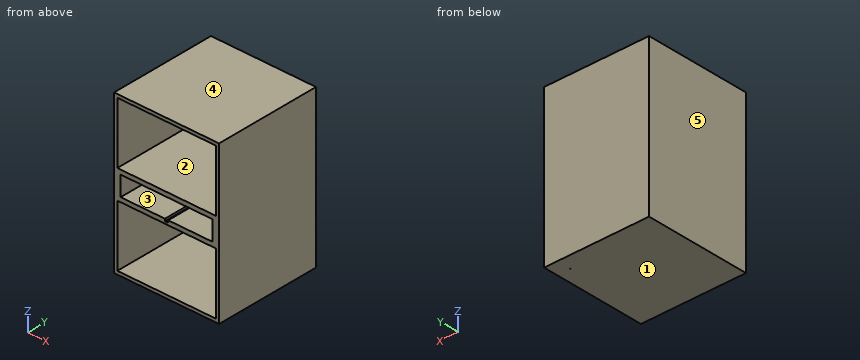
from build123d import *

# Parameters (mm, degrees)
F0_W     = 1219.2
F0_H     = 1828.8
F0_W_2   = 1143
F0_H_2   = 711.2
F0_W_3   = 1066.8
F0_H_3   = 228.6
F1_DEPTH = 609.6
F2_W     = 1219.2
F2_H     = 1828.8
F3_DEPTH = 12.7
F5_D     = 2.54
F7_D     = 2.54
F7_DEPTH = 12.7
F7_TIP   = 0.7630929862
F8_W     = 38.1
F8_H     = 1219.2
F9_DEPTH = 25.4


# Not quite as in the source:
# - a feature names something its author has since deleted; it is built from what else it names


with BuildPart() as f1:
    # F0 (on Front) → F1 (new body, symmetric)
    with BuildSketch(Plane.XZ):
        Rectangle(F0_W, F0_H)
        with Locations((0, -520.7)):
            Rectangle(F0_W_2, F0_H_2, mode=Mode.SUBTRACT)
        Rectangle(F0_W_3, F0_H_3, mode=Mode.SUBTRACT)
        with Locations((0, 520.7)):
            Rectangle(F0_W_2, F0_H_2, mode=Mode.SUBTRACT)
    extrude(amount=F1_DEPTH, both=True)

    # F2 (on face) → F3 (join)
    with BuildSketch(Plane(origin=(0, 609.6, 0), x_dir=(-1, 0, 0), z_dir=(0, 1, 0))):
        Rectangle(F2_W, F2_H)
    extrude(amount=F3_DEPTH)

    # F5 (through all)
    with Locations(Plane(origin=(-609.6, 0, 0), x_dir=(0, -1, 0), z_dir=(-1, 0, 0))):
        with Locations((-400.05, 685.8), (-311.15, 685.8), (311.15, 685.8), (400.05, 685.8)):
            Hole(F5_D / 2)

    # F7
    with Locations(Plane(origin=(0, 0, -914.4), x_dir=(1, 0, 0), z_dir=(0, 0, -1))):
        with Locations((-457.2, 457.2), (457.2, 457.2), (457.2, -457.2), (-457.2, -457.2)):
            Hole(F7_D / 2, depth=F7_DEPTH)
            with Locations((0, 0, -(F7_DEPTH + F7_TIP / 2))):  # 118° drill point
                Cone(0, F7_D / 2, F7_TIP, mode=Mode.SUBTRACT)

    # F8 (on face) → F9 (cut)
    with BuildSketch(Plane.XY.offset(-114.3)):
        Rectangle(F8_W, F8_H)
    extrude(amount=-F9_DEPTH, mode=Mode.SUBTRACT)


solid = f1.part
Design review of the part built by this model. Coordinates are the model's own, in mm. Face numbers are marked on the shaded views. A direction names the side the tool comes from. Round coordinates to 2 decimals unless told otherwise and drop trailing zeros. Loops run counter-clockwise (first coordinate to the right, second up) from the corner with the lowest first, then second, coordinate; pieces in that order, holes last. Notation, with made-up numbers: M -24.75,89.25 L -1.75,89.25 A20 cw -1.75,117.25 Z; hole C 12,14 d8. An arc over 180 degrees is marked long. Answer as a JSON object with one key per item and string values.
Item 1: Machinability: for the marked faces 1 and 2, which of the approach directions +Z, -Z, +X, -X, +Y, -Y give a long, thin tool a straight path to every point of the face, cutting with its end or side? Answer none if there is none.
Answer sheet:
{"face 1": "-Z, +X, -X, +Y, -Y", "face 2": "-Y"}
Item 2: Clearance check with flat-ended pins moving along their axes: P1, Ø1.5, axis at y = -311.15, z = 685.8, coming from the +X side; P2, Ø2, axis at x = 457.2, y = -457.2, coming from the -Z side. State where each tip first meets the part, or that it passes through.
Answer sheet:
{"P1": "passes through", "P2": "stops at z = -901.54"}
Item 3: We need section A-A on z = 9.5. Give the boundary of the cut face in (x, y), and give its area (3 significant figures).
Answer sheet:
{"outline": "M -609.6,-609.6 L -533.4,-609.6 L -533.4,609.6 L 533.4,609.6 L 533.4,-609.6 L 609.6,-609.6 L 609.6,622.3 L -609.6,622.3 Z", "area": "201,000 mm^2"}
Item 4: The part is to be moulded in two halves that separate along X. For the marked faces 3, 4 and 5, say which applies: pulls with the +X half, pulls with the -X half, needs draft (parallel to the pull), parting line crosses it, or undercut.
Answer sheet:
{"face 3": "undercut", "face 4": "needs draft", "face 5": "pulls with the -X half"}
Item 5: We need section C-C on x = -506. Give the boundary of the cut face in (y, z).
Answer sheet:
{"outline": "M -609.6,-914.4 L 622.3,-914.4 L 622.3,914.4 L -609.6,914.4 L -609.6,876.3 L 609.6,876.3 L 609.6,165.1 L -609.6,165.1 L -609.6,114.3 L 609.6,114.3 L 609.6,-114.3 L -609.6,-114.3 L -609.6,-165.1 L 609.6,-165.1 L 609.6,-876.3 L -609.6,-876.3 Z"}
Item 6: We need section B-B on y = 261. Give the boundary of the cut face in (x, z), and give its area (3 significant figures).
Answer sheet:
{"outline": "M -609.6,-914.4 L 609.6,-914.4 L 609.6,914.4 L -609.6,914.4 Z; hole M -571.5,-876.3 L 571.5,-876.3 L 571.5,-165.1 L -571.5,-165.1 Z; hole M -571.5,165.1 L 571.5,165.1 L 571.5,876.3 L -571.5,876.3 Z; hole M -533.4,-114.3 L -19.05,-114.3 L -19.05,-139.7 L 19.05,-139.7 L 19.05,-114.3 L 533.4,-114.3 L 533.4,114.3 L -533.4,114.3 Z", "area": "359,000 mm^2"}
Item 7: Wall thickness on L1, parallel to Z at x = -323, y = -252; L2, parallel to Y at x = -598, z = 685; L3, parallel to Y at x = 457, z = -910: over which ranges is each line inside the solid? List them lowest first. Write a range as from..to.
Answer sheet:
{"L1": "z = -914.4..-876.3, -165.1..-114.3, 114.3..165.1, 876.3..914.4", "L2": "y = -609.6..-401.04, -399.06..-312.14, -310.16..310.16, 312.14..399.06, 401.04..622.3", "L3": "y = -609.6..-458.45, -455.95..455.95, 458.45..622.3"}
Item 8: We need section D-D on z = 602. Give the boundary of the cut face in (x, y), and give its area (3 significant figures).
Answer sheet:
{"outline": "M -609.6,-609.6 L -571.5,-609.6 L -571.5,609.6 L 571.5,609.6 L 571.5,-609.6 L 609.6,-609.6 L 609.6,622.3 L -609.6,622.3 Z", "area": "108,000 mm^2"}
